The listing builds one solid part. Answer for the finished solid, in the listing's coordinates (mm). Round coordinates to 2 decimals unless told otherwise and drop trailing zeros. Order: outer loops, then holes, each group sorted by start corner. A loop starts at its lowest first (then second) coordinate and runs counter-clockwise, first axis right, second up. Notation, with made-up numbers: (-24, 83) - (-15, 83) arc R24 ccw to (-15, 93) - close; hole circle Ø3 at (51.5, -13.5). An arc over 180 degrees is marked (long way). One line per item, written item: value. Start each with the question number.
1. Section A-A, the plane z = -38 is taken. Give the vertices of the cut face in (x, y), then the cut area to 3 significant figures.
2. Section B-B, the plane x = 52.5 is taken. Give the vertices of the cut face in (y, z), then the cut area to 3 significant figures.
3. Section C-C, the plane y = 12 is taken. Give the vertices of the cut face in (x, z), then the cut area to 3 significant figures.
4. Section D-D, the plane z = -16 is taken. Count the separate pieces of the cut face and the enclosed holes in it, then the cut area to 3 significant figures.
5. A flat-ended cylindrical pin translates along its axis: P1, Ø3, axis at x = 28, z = 30.5, coming from the +Y side. Find the tip coordinate at first contact, or state that the pin passes through.
6. Straight lines are drawn through the part: line 1 (Z direction, x = 52.5, y = 0.85); line 2 (Y direction, x = -20.5, z = -29.5); line 3 (Z direction, x = -2, y = 1.25). For each, find the intervals that lie inside material, in ascending order.
Autodesk Inventor part; units mm, degrees
ref_plane "YZ Plane" through (0, 0, 0) normal (1, 0, 0) x (0, 1, 0)
ref_plane "XZ Plane" through (0, 0, 0) normal (0, 1, 0) x (-1, 0, 0)
ref_plane "XY Plane" through (0, 0, 0) normal (0, 0, 1) x (1, 0, 0)
sketch "Szkic1" plane through (0, 0, 0) normal (0, 1, 0) x (-1, 0, 0)
  line L0 (58.5, -44) -> (-58.5, -44)
  line L1 (-58.5, -44) -> (-58.5, 44)
  line L2 (-58.5, 44) -> (58.5, 44)
  line L3 (58.5, 44) -> (58.5, -44)
  line L4 (58.5, -44) -> (-58.5, 44) construction
  line L5 (-58.5, -44) -> (58.5, 44) construction
  point P0 (0, 0)
  dimension "d0" = 117
  dimension "d1" = 88
extrude "Wyciągnięcie proste1" add sketch "Szkic1" along normal blind 1.2
sketch "Szkic2" plane through (0, 1.2, 0) normal (0, 1, 0) x (1, 0, 0)
  line L0 (-52.5, 38) -> (-52.5, 44)
  line L1 (58.5, 44) -> (-58.5, 44)
  line L2 (-52.5, 38) -> (-46.5, 38) construction
  line L3 (-52.5, 38) -> (-58.5, 38)
  line L4 (-58.5, 44) -> (-58.5, -44)
  line L5 (-52.5, 38) -> (-46.5, 38) construction
  circle A0 centre (-52.5, 38) radius 2
  point P0 (0, 0)
  dimension "d4" = 6
  dimension "d5" = 90
  dimension "d6" = 6
  dimension "d7" = 180
  dimension "d8" = 4
extrude "Wyciągnięcie proste2" cut sketch "Szkic2" against normal through all contours L3 A0 L0 | L0 A0 L3
mirror "Odbij1" about plane through (0, 0, 0) normal (0, 0, 1) of "Wyciągnięcie proste2"
mirror "Odbij2" about plane through (0, 0, 0) normal (1, 0, 0) of "Wyciągnięcie proste2", "Odbij1"
sketch "Szkic3" plane through (0, 1.2, 0) normal (0, 1, 0) x (1, 0, 0)
  line L0 (-2.5, -34) -> (-58.5, -34)
  line L1 (-2.5, -34) -> (53.5, -34) construction
  line L2 (-2.5, -34) -> (-2.5, -44)
  line L3 (-2.5, -34) -> (7.5, -34) construction
  line L4 (-58.5, 44) -> (-58.5, -44)
  line L5 (-58.5, -44) -> (58.5, -44)
  circle A0 centre (-2.5, -34) radius 2
  line L6 (-2.5, -34) -> (-2.5, -12)
  line L7 (-2.5, -34) -> (19.5, -34) construction
  circle A1 centre (-2.5, -12) radius 2
  point P0 (0, 0)
  dimension "d11" = 56
  dimension "d12" = 180
  dimension "d13" = 10
  dimension "d14" = 90
  dimension "d15" = 4
  dimension "d16" = 22
  dimension "d17" = 90
  dimension "d18" = 4
extrude "Wyciągnięcie proste3" add sketch "Szkic3" along normal blind 2 contours L2 A0 L0 | L6 A0 L2 | L0 A0 L6 | A1
sketch "Szkic4" plane through (-2.5, 3.2, 34) normal (0, 1, 0) x (1, 0, 0)
  circle A0 centre (0, 0) radius 1
  circle A1 centre (0, 22) radius 2
  circle A2 centre (0, 22) radius 1
  point P0 (2.5, 34)
  dimension "d21" = 2
  dimension "d22" = 2
extrude "Wyciągnięcie proste4" add sketch "Szkic4" along normal blind 4 contours A0 | A2
sketch "Szkic5" plane through (0, 1.2, 0) normal (0, 1, 0) x (1, 0, 0)
  line L0 (1.5, -4) -> (3.1, -4)
  line L1 (3.1, -4) -> (3.1, -39)
  line L2 (3.1, -39) -> (1.5, -39)
  line L3 (1.5, -39) -> (1.5, -4)
  line L4 (2.3, -39) -> (2.3, -44)
  line L5 (-58.5, -44) -> (58.5, -44)
  line L6 (1.5, -15.8672) -> (-58.5, -15.8672)
  line L7 (-58.5, 44) -> (-58.5, -44)
  point P0 (0, 0)
  dimension "d25" = 1.6
  dimension "d26" = 35
  dimension "d27" = 5
  dimension "d28" = 60
extrude "Wyciągnięcie proste5" add sketch "Szkic5" along normal blind 14 contours L0 L1 L2 L3
sketch "Szkic6" plane through (0, 1.2, 0) normal (0, 1, 0) x (1, 0, 0)
  line L0 (3.1, -4) -> (1.5, -4)
  line L1 (1.5, -4) -> (-2.5, -4)
  line L2 (-2.5, -4) -> (-2.5, -5.2)
  line L3 (-2.5, -5.2) -> (1.5, -5.2)
  line L4 (1.5, -5.2) -> (1.5, -4)
  point P0 (0, 0)
  dimension "d31" = 4
  dimension "d32" = 1.2
extrude "Wyciągnięcie proste6" add sketch "Szkic6" along normal blind 14
sketch "Szkic7" plane through (0, 1.2, 0) normal (0, 1, 0) x (1, 0, 0)
  line L0 (-47, 32) -> (-43, 32)
  line L1 (-43, 32) -> (-43, 2)
  line L2 (-43, 2) -> (-47, 2)
  line L3 (-47, 2) -> (-47, 32)
  line L4 (-47, 28.7975) -> (-58.5, 28.7975)
  line L5 (-47, 28.7975) -> (-35.5, 28.7975) construction
  line L6 (-58.5, 44) -> (-58.5, -44)
  line L7 (-45, 32) -> (-45, 44)
  line L8 (-45, 32) -> (-33, 32) construction
  line L9 (58.5, 44) -> (-58.5, 44)
  point P0 (0, 0)
  dimension "d35" = 4
  dimension "d36" = 30
  dimension "d37" = 11.5
  dimension "d38" = 180
  dimension "d39" = 12
  dimension "d40" = 90
extrude "Wyciągnięcie proste7" cut sketch "Szkic7" against normal through all contours L0 L1 L2 L3
pattern_linear "Szyk prostokątny3" count 10 spacing 10 along (1, 0, 0) of "Wyciągnięcie proste7"
mirror "Odbij5" about plane through (0, 0, 0) normal (0, 0, 1) of "Wyciągnięcie proste7", "Szyk prostokątny3"
sketch "Szkic8" plane through (0, 1.2, 0) normal (0, 1, 0) x (1, 0, 0)
  line L0 (-7, -32) -> (-7, -2)
  line L1 (7, -2) -> (-7, -2)
  line L2 (-7, -2) -> (-7, -32)
  line L3 (-7, -32) -> (7, -32)
  line L4 (7, -32) -> (7, -2)
  point P0 (0, 0)
  point P1 (-7, -2)
extrude "Wyciągnięcie proste8" add sketch "Szkic8" against normal up to surface (1.2 mm away)
properties part number "platforma"
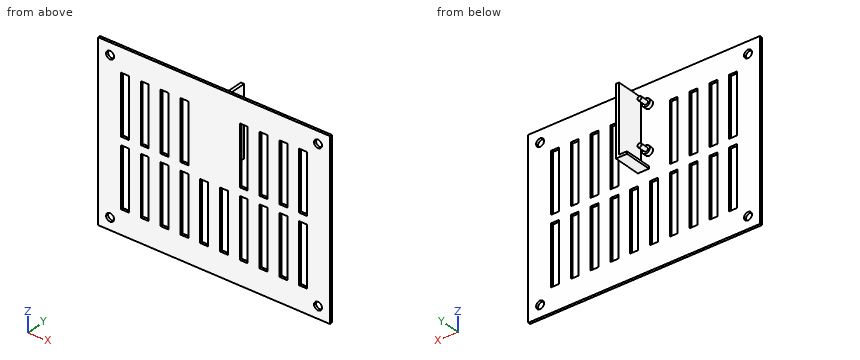
Answer list:
1. outline: (-58.5, 0) - (-54.5, 0) - (-54.5, 1.2) - (-58.5, 1.2) - close; (-50.5, 0) - (50.5, 0) - (50.5, 1.2) - (-50.5, 1.2) - close; (54.5, 0) - (58.5, 0) - (58.5, 1.2) - (54.5, 1.2) - close
1. area: 131 mm²
2. outline: (0, -44) - (1.2, -44) - (1.2, -40) - (0, -40) - close; (0, -36) - (1.2, -36) - (1.2, 36) - (0, 36) - close; (0, 40) - (1.2, 40) - (1.2, 44) - (0, 44) - close
2. area: 96.0 mm²
3. outline: (-2.5, 4) - (3.1, 4) - (3.1, 39) - (1.5, 39) - (1.5, 5.2) - (-2.5, 5.2) - close
3. area: 60.8 mm²
4. separate pieces: 11
4. enclosed holes: 0
4. area: 92.4 mm²
5. P1: stops at y = 1.2
6. line 1: z = -44 to -40, -36 to 36, 40 to 44
6. line 2: y = 0 to 1.2
6. line 3: z = 4 to 5.2, 10.06 to 13.94, 32.06 to 35.94
